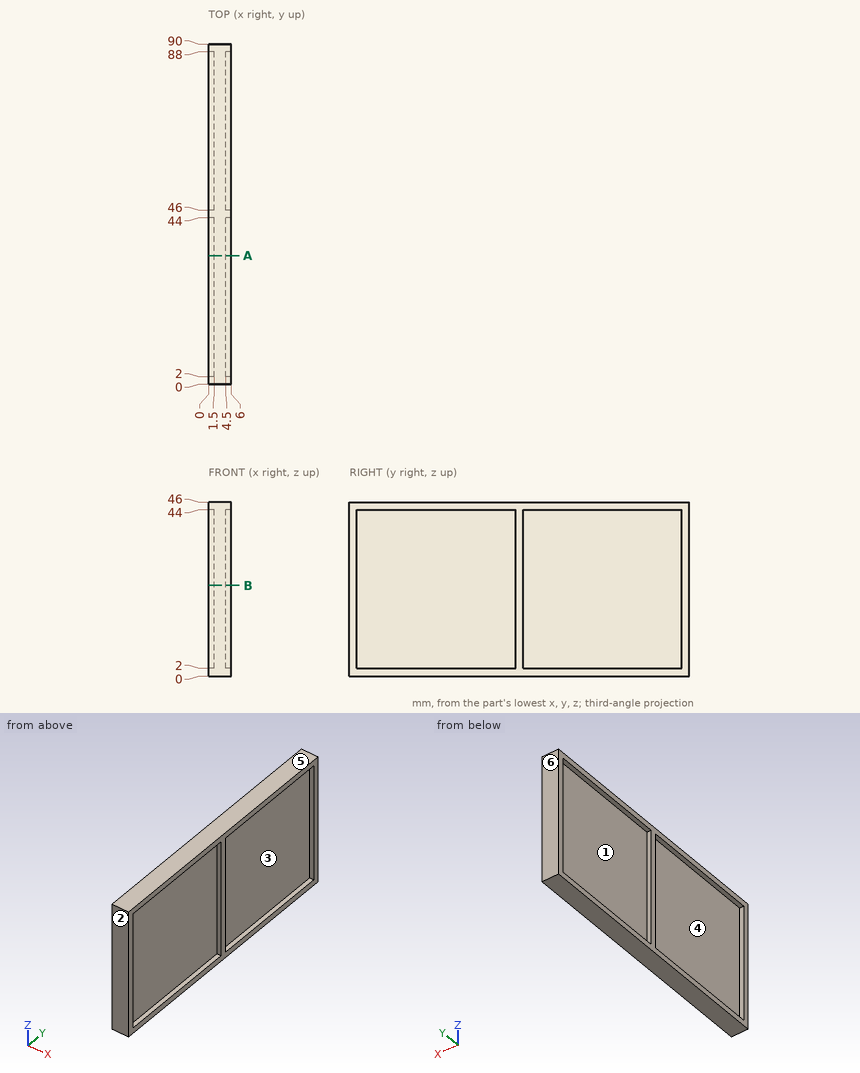
Verification items for this drawing (mm, ordinates from the low corner). A direction names the side the tool comes from. Coordinates: 2 decimals unless noted, no trailing zeros. Order: outer loops, then holes, each group sorted by start corner. A loop starts at its lowest first (then second) coordinate and runs counter-clockwise, first axis right, second up. Notation, with made-up numbers: M 0,-26 L 48,-26 A19 cw 48,0 Z; hole C 8.25,43.25 d6. An arc over 180 degrees is marked long. One line per item, written item: value. Start each with the question number.
Item 1: Mould release check, pull along Y, two halves, no side actions. Record for the marked faces 4, 5 and 6: pulls with the +Y half, pulls with the -Y half, needs draft (parallel to the pull), parting line crosses it, or undercut.
Item 2: Sectioned sample at A-A on y = 34. Record the cut outline in (x, z).
Item 3: Sectioned sample at B-B on z = 24. Record the cut outline in (x, y).
Item 4: Access from +Z, -Z, +X, -X, +Y, -Y to the whole of each face (thin tool, end or side, straight path). Record for the marked faces 1, 2 and 3.
Item 5: Thickness scan on probe 1 along Y at (x, z) = (0.55, 32.5); probe 2 along Z at (x, y) = (5.45, 23); probe 3 along X at (y, z) = (13.5, 37). Record the ranges inside material, lowest first.
Item 6: Depth check by flat-ended pin: P1, Ø8, axis at y = 68, z = 6.5, coming from the -X side. Enter the tip coordinate at first touch or a pass-through.
Calculated:
1. face 4: undercut
1. face 5: needs draft
1. face 6: pulls with the +Y half
2. outline: M 0,0 L 6,0 L 6,2 L 4.5,2 L 4.5,44 L 6,44 L 6,46 L 0,46 L 0,44 L 1.5,44 L 1.5,2 L 0,2 Z
3. outline: M 0,0 L 6,0 L 6,2 L 4.5,2 L 4.5,44 L 6,44 L 6,46 L 4.5,46 L 4.5,88 L 6,88 L 6,90 L 0,90 L 0,88 L 1.5,88 L 1.5,46 L 0,46 L 0,44 L 1.5,44 L 1.5,2 L 0,2 Z
4. face 1: -X
4. face 2: +Z, -Z, +X, -X, -Y
4. face 3: +X
5. probe 1: 0 to 2, 44 to 46, 88 to 90
5. probe 2: 0 to 2, 44 to 46
5. probe 3: 1.5 to 4.5
6. P1: x = 1.5
